from build123d import *

# Parameters (mm, degrees)
SKETCH1_W                                      = 304.8
SKETCH1_H                                      = 152.4
BOSS_EXTRUDE1_DEPTH                            = 11.1125
CUT_EXTRUDE1_DEPTH                             = 11.1125
CUT_EXTRUDE2_REACH                             = 143.224
SKETCH5_W                                      = 24.13
SKETCH5_H                                      = 2.677814457
SKETCH5_H_2                                    = 2.54
CBORE_FOR_8_SOCKET_HEAD_CAP_SCREW1_D           = 4.3053
CBORE_FOR_8_SOCKET_HEAD_CAP_SCREW1_DEPTH       = 11.1125
CBORE_FOR_8_SOCKET_HEAD_CAP_SCREW1_CBORE_D     = 7.9375
CBORE_FOR_8_SOCKET_HEAD_CAP_SCREW1_CBORE_DEPTH = 4.1656
CBORE_FOR_8_SOCKET_HEAD_CAP_SCREW3_D           = 4.3053
CBORE_FOR_8_SOCKET_HEAD_CAP_SCREW3_DEPTH       = 11.1125
CBORE_FOR_8_SOCKET_HEAD_CAP_SCREW3_CBORE_D     = 7.9375
CBORE_FOR_8_SOCKET_HEAD_CAP_SCREW3_CBORE_DEPTH = 4.1656


with BuildPart() as part:
    # Sketch1 → Boss-Extrude1 (new body)
    with BuildSketch(Plane(origin=(0, 0, 0), x_dir=(1, 0, 0), z_dir=(0, 1, 0))):
        with Locations((152.4, 76.2)):
            Rectangle(SKETCH1_W, SKETCH1_H)
    extrude(amount=BOSS_EXTRUDE1_DEPTH)

    # Sketch3 → Cut-Extrude1 (cut)
    with BuildSketch(Plane(origin=(0, 11.1125, 0), x_dir=(1, 0, 0), z_dir=(0, 1, 0))):
        with BuildLine():
            Line((280.86812, 11.176), (256.73812, 11.176))
            ThreePointArc((256.73812, 11.176), (254.32512, 8.763), (256.73812, 6.35))
            Line((256.73812, 6.35), (280.86812, 6.35))
            ThreePointArc((280.86812, 6.35), (283.28112, 8.763), (280.86812, 11.176))
        make_face()
        with BuildLine():
            Line((280.86812, 97.9932), (256.73812, 97.9932))
            ThreePointArc((256.73812, 97.9932), (254.32512, 95.5802), (256.73812, 93.1672))
            Line((256.73812, 93.1672), (280.86812, 93.1672))
            ThreePointArc((280.86812, 93.1672), (283.28112, 95.5802), (280.86812, 97.9932))
        make_face()
        with BuildLine():
            Line((212.54212, 97.9932), (188.41212, 97.9932))
            ThreePointArc((188.41212, 97.9932), (185.99912, 95.5802), (188.41212, 93.1672))
            Line((188.41212, 93.1672), (212.54212, 93.1672))
            ThreePointArc((212.54212, 93.1672), (214.95512, 95.5802), (212.54212, 97.9932))
        make_face()
        with BuildLine():
            ThreePointArc((212.54212, 6.35), (214.95512, 8.763), (212.54212, 11.176))
            Line((212.54212, 11.176), (188.41212, 11.176))
            ThreePointArc((188.41212, 11.176), (185.99912, 8.763), (188.41212, 6.35))
            Line((188.41212, 6.35), (212.54212, 6.35))
        make_face()
    extrude(amount=-CUT_EXTRUDE1_DEPTH, mode=Mode.SUBTRACT)

    # Sketch5 → Cut-Extrude2 (cut, up to next)
    with BuildSketch(Plane.XY.offset(-11.176), mode=Mode.PRIVATE) as cut_extrude2_sk1:
        with Locations((200.47712, 1.338907229)):
            Rectangle(SKETCH5_W, SKETCH5_H)
    cut_extrude2_tool1 = extrude(cut_extrude2_sk1.sketch, amount=-CUT_EXTRUDE2_REACH, mode=Mode.PRIVATE) & part.part
    add(cut_extrude2_tool1.solids().sort_by_distance((200.47712, 1.338907, -11.176))[0], mode=Mode.SUBTRACT)
    # Sketch5 → Cut-Extrude2 (cut, up to next)
    with BuildSketch(Plane.XY.offset(-11.176), mode=Mode.PRIVATE) as cut_extrude2_sk2:
        with Locations((268.80312, 1.27)):
            Rectangle(SKETCH5_W, SKETCH5_H_2)
    cut_extrude2_tool2 = extrude(cut_extrude2_sk2.sketch, amount=-CUT_EXTRUDE2_REACH, mode=Mode.PRIVATE) & part.part
    add(cut_extrude2_tool2.solids().sort_by_distance((268.80312, 1.27, -11.176))[0], mode=Mode.SUBTRACT)

    # CBORE for #8 Socket Head Cap Screw1
    with Locations(Plane(origin=(161.6075, 0, -13.516787713), x_dir=(0, 0, -1), z_dir=(0, -1, 0))):
        with Locations((0, 0), (0, -18.415), (77.309624574, 0), (77.309624574, -18.415)):
            CounterBoreHole(CBORE_FOR_8_SOCKET_HEAD_CAP_SCREW1_D / 2, CBORE_FOR_8_SOCKET_HEAD_CAP_SCREW1_CBORE_D / 2, CBORE_FOR_8_SOCKET_HEAD_CAP_SCREW1_CBORE_DEPTH, depth=CBORE_FOR_8_SOCKET_HEAD_CAP_SCREW1_DEPTH)

    # CBORE for #8 Socket Head Cap Screw3
    with Locations(Plane(origin=(95.25, 0, -39.4716), x_dir=(0, 0, -1), z_dir=(0, -1, 0))):
        with Locations((0, 0), (25.4, 0), (0, -38.1), (25.4, -38.1), (0, -76.2), (25.4, -76.2)):
            CounterBoreHole(CBORE_FOR_8_SOCKET_HEAD_CAP_SCREW3_D / 2, CBORE_FOR_8_SOCKET_HEAD_CAP_SCREW3_CBORE_D / 2, CBORE_FOR_8_SOCKET_HEAD_CAP_SCREW3_CBORE_DEPTH, depth=CBORE_FOR_8_SOCKET_HEAD_CAP_SCREW3_DEPTH)


solid = part.part
Source: CAD feature listing. Evaluate the final solid. Frame: model axes, mm. A direction names the side the tool comes from. Give positions to 0.01 mm unless a question says otherwise; leave off trailing zeros. Write each loop counter-clockwise with the first axis right and the second up, starting at its lowest first coordinate (ties: lowest second). Pieces come first, ordered by that corner, then holes. Notation, with made-up numbers: (-3.5, 51) -> (35.5, 51) arc R37 cw to (35.5, 89) -> close; hole circle Ø7 at (62.5, -29). An arc over 180 degrees is marked (long way). Return JSON: item names as keys, results as strings. Group by question number.
1. Mould query, pull axis Z, two halves, no side actions, for faces 3 (the face through (150, 11.112, -77)), 4 (the face through (19.224, 2.054, -60.907)). Classes: +Z half, -Z half, draft (parallel to the pull), parting line (faces both ways), or undercut.
2. Section A-A, the plane z = -51. Output: boundary loops of the cut face in (x, y), then the cut area to 3 significant figures.
3. Material intervals for line 1 (Z direction, x = 265.5, y = 10.75); line 2 (X direction, y = 1.5, z = -58); line 3 (Z direction, x = 161.5, y = 6), sorted ascending. Write a range as from..to.
4. Access query for faces 1 (the face through (269, 7, -11.176)), 2 (the face through (54.74, 2.05, -36.32)). Directions: +Z, -Z, +X, -X, +Y, -Y. A direction counts if a zero-diameter tool reaches every point of the face in a straight line with its end or side. Return the directions, or none.
5. Pin query (flat end, axial travel): pin 1 Ø4 at (x, z) = (96, -66.5) entering from -Y; pin 2 Ø2.5 at (x, y) = (272, 7.5) entering from +Z; pin 3 Ø12 at (x, z) = (196, -60.5) entering from -Y. Return the tip coordinate at first contact, or that it passes through.
Determined:
{
 "1": {"face 3": "draft", "face 4": "undercut"},
 "2": {"outline": "(0, 0) -> (188.41, 0) -> (188.41, 2.68) -> (212.54, 2.68) -> (212.54, 0) -> (256.74, 0) -> (256.74, 2.54) -> (280.87, 2.54) -> (280.87, 0) -> (304.8, 0) -> (304.8, 11.11) -> (0, 11.11) -> close", "area": "3,260 mm2"},
 "3": {"line 1": "z = -152.4..-97.99, -93.17..-11.18, -6.35..0", "line 2": "x = 0..188.41, 212.54..256.74, 280.87..304.8", "line 3": "z = -152.4..-92.98, -88.68..-15.67, -11.37..0"},
 "4": {"face 1": "+Y, -Y", "face 2": "-Y"},
 "5": {"pin 1": "stops at y = 4.17", "pin 2": "stops at z = 0", "pin 3": "stops at y = 2.68"}
}
